from build123d import *

# Parameters (mm, degrees)
SKETCH1_W               = 90.621510256
SKETCH1_H               = 47.057987938
BOSS_EXTRUDE1_DEPTH     = 23.009727366
BOSS_EXTRUDE3_START     = -90.621510256
BOSS_EXTRUDE3_OUTLINE_R = 5
BOSS_EXTRUDE3_DEPTH     = 90.621510256
SKETCH11_R              = 5
CUT_EXTRUDE3_DEPTH      = 19.832993722
CIRPATTERN1_COUNT       = 2
CIRPATTERN2_START       = -23.009727366
CIRPATTERN2_OUTLINE_R   = 5
CIRPATTERN2_DEPTH       = 19.832993722


# Read off the part's stored shape, not the designer's step: Boss-Extrude3, CirPattern2
with BuildPart() as part:
    # Sketch1 → Boss-Extrude1 (new body)
    with BuildSketch(Plane.XY):
        Rectangle(SKETCH1_W, SKETCH1_H)
    extrude(amount=BOSS_EXTRUDE1_DEPTH)

    # Boss-Extrude3 outline → Boss-Extrude3 (cut)
    with BuildSketch(Plane(origin=(45.310755128, 0, 0), x_dir=(0, 0, -1), z_dir=(1, 0, 0)).offset(BOSS_EXTRUDE3_START)):
        with Locations((-13.009727366, 13.528993969)):
            Circle(BOSS_EXTRUDE3_OUTLINE_R)
    boss_extrude3 = extrude(amount=BOSS_EXTRUDE3_DEPTH, mode=Mode.SUBTRACT)

    # Mirror4: Boss-Extrude3 across plane
    add(boss_extrude3.mirror(Plane.ZX), mode=Mode.SUBTRACT)

    # Mirror5: part across plane


with BuildPart() as part_1:
    add(part.part)
    add(part.part.mirror(Plane.XY))

    # Sketch11 → Cut-Extrude3 (cut)
    with BuildSketch(Plane.XY.offset(23.009727366)):
        with Locations((-35.310755128, 13.528993969)):
            Circle(SKETCH11_R)
    cut_extrude3 = extrude(amount=-CUT_EXTRUDE3_DEPTH, mode=Mode.SUBTRACT)

    # CirPattern1: Cut-Extrude3 ×2 about axis
    cirpattern1_axis = Axis((0.662529663, -0.253842201, 0), (0, 0, 1))
    for i in range(1, CIRPATTERN1_COUNT):
        add(cut_extrude3.rotate(cirpattern1_axis, i * 360 / CIRPATTERN1_COUNT), mode=Mode.SUBTRACT)

    # CirPattern2 outline → CirPattern2 (cut)
    with BuildSketch(Plane.XY.offset(CIRPATTERN2_START)):
        with Locations((-35.310755128, -13.528993969)):
            Circle(CIRPATTERN2_OUTLINE_R)
        with Locations((35.260080607, 13.509578489)):
            Circle(CIRPATTERN2_OUTLINE_R)
    extrude(amount=CIRPATTERN2_DEPTH, mode=Mode.SUBTRACT)


solid = part_1.part
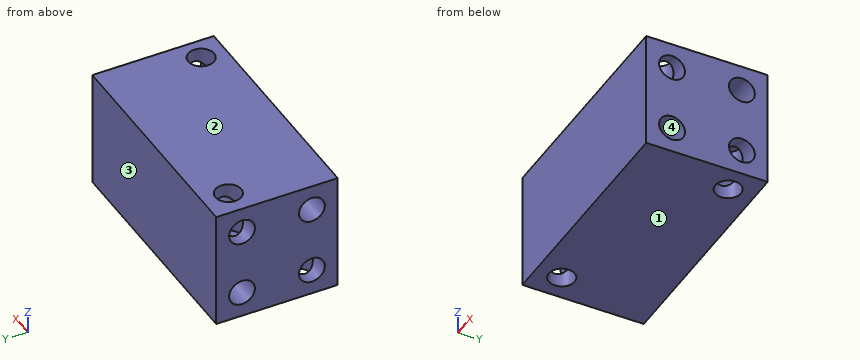
Build history of the part. All positions in model axes, mm. Face numbers are marked on the shaded views. Coordinates: 2 decimals unless noted, no trailing zeros. Write each loop counter-clockwise with the first axis right and the second up, starting at its lowest first coordinate (ties: lowest second). Pieces come first, ordered by that corner, then holes. Notation, with made-up numbers: (68.25, -7.5) -> (77.25, -7.5) arc R13 ccw to (77.25, 10.5) -> close; hole circle Ø3 at (9, 66.25). An arc over 180 degrees is marked (long way). Use CSV: the item, a comma, the result in double quotes. Start each with the question number.
Q1. Cut at A-A, the plane x = -33. List the corners of the cut face in (y, z).
Q2. Cut at B-B, the plane x = -5. List the corners of the cut face in (y, z), then the cut area to 3 significant figures.
Q3. Drill centre lines: probe 1 along X at (y, z) = (-14, -21); probe 2 along Y at (x, z) = (20.5, -16); probe 3 along Z at (x, y) = (20, -16.5). Where is each one in solid material? Low to high.
Q4. Pull direction Z, two halves, no side cores. Call the marked faces 1, 2, 3 and 4: released by +Z, released by -Z, zero draft, split by the parting line, or undercut.
Q5. Cut at C-C, the plane z = 5. List the corners of the cut face in (x, y), then the cut area to 3 significant figures.
Q6. Flat gauge pins, fed straight in: pin 1 Ø5 at (x, y) = (-35, -13.5) entering from -Z; pin 2 Ø3 at (x, y) = (34, -12.5) entering from +Z. Where does each tip first touch, or does it go through?
Checked values:
1,outline,"(-23.53, -23.01) -> (-17.96, -23.01) -> (-17.96, -15.32) arc R5 cw to (-17.96, -10.7) -> (-17.96, -3.18) -> (-9.09, -3.18) -> (-9.09, -10.7) arc R5 cw to (-9.09, -15.32) -> (-9.09, -23.01) -> (23.53, -23.01) -> (23.53, 23.01) -> (17.96, 23.01) -> (17.96, 15.32) arc R5 cw to (17.96, 10.7) -> (17.96, 3.18) -> (9.09, 3.18) -> (9.09, 10.7) arc R5 cw to (9.09, 15.32) -> (9.09, 23.01) -> (-23.53, 23.01) -> close; hole circle Ø10 at (-13.53, 13.01); hole circle Ø10 at (13.53, -13.01)"
2,outline,"(-23.53, -23.01) -> (23.53, -23.01) -> (23.53, 23.01) -> (-23.53, 23.01) -> close; hole circle Ø10 at (-13.53, -13.01); hole circle Ø10 at (-13.53, 13.01); hole circle Ø10 at (13.53, -13.01); hole circle Ø10 at (13.53, 13.01)"
2,area,"1,850 mm²"
3,probe 1,"x = -45.31 to -40.29, -30.33 to 45.31"
3,probe 2,"y = -23.53 to -17.54, -9.52 to 9.52, 17.54 to 23.53"
3,probe 3,"z = -23.01 to -17.03, -8.99 to 8.99, 17.03 to 23.01"
4,face 1,"released by -Z"
4,face 2,"released by +Z"
4,face 3,"zero draft"
4,face 4,"undercut"
5,outline,"(-45.31, -23.53) -> (45.31, -23.53) -> (45.31, 23.53) -> (-45.31, 23.53) -> close; hole circle Ø10 at (-35.31, 13.53); hole circle Ø10 at (36.64, -14.04)"
5,area,"4,110 mm²"
6,pin 1,"stops at z = -3.18"
6,pin 2,"stops at z = 3.18"
